```python
from build123d import *

# Parameters (mm, degrees)
FILLET1_R           = 1
SKETCH3_R           = 5.5
CUT_EXTRUDE1_DEPTH  = 0.35
CUT_EXTRUDE2_DEPTH  = 5
BOSS_EXTRUDE2_DEPTH = 2
SKETCH5_R           = 0.65
CUT_EXTRUDE3_DEPTH  = 5
SKETCH7_R           = 1.1
CUT_EXTRUDE4_DEPTH  = 8


with BuildPart() as part:
    # Sketch1 → Revolve1 (revolve)
    with BuildSketch(Plane.XY, mode=Mode.PRIVATE) as revolve1_sk:
        Polygon((-17.325922144, -3.94739572), (34.674077856, -3.94739572), (34.674077856, -4.54739572), (-17.825922144, -4.54739572), (-18.531230067, -0.94739572), (-18.531230067, 0.05260428), (-18.031230067, 0.05260428), align=None)
    revolve(revolve1_sk.sketch.rotate(Axis((-18.92728318, 4.55260428, 0), (1, 0, 0)), 270), axis=Axis((-18.92728318, 4.55260428, 0), (1, 0, 0)))

    # Fillet1
    fillet1_edges = [part.edges().sort_by_distance(p)[0] for p in [
        (-17.825922144, 4.55260428, -9.1),
    ]]
    fillet(fillet1_edges, radius=FILLET1_R)

    # Sketch3 → Cut-Extrude1 (cut)
    with BuildSketch(Plane.ZY.offset(18.531230067)):
        with Locations((0, 4.55260428)):
            Circle(SKETCH3_R)
    extrude(amount=-CUT_EXTRUDE1_DEPTH, mode=Mode.SUBTRACT)

    # Sketch4 → Cut-Extrude2 (cut)
    with BuildSketch(Plane(origin=(34.674077856, 0, 0), x_dir=(0, 0, -1), z_dir=(1, 0, 0))):
        Polygon((-13.628095951, 5.995190129), (5.056342646, -9.067736356), (14.470671699, 2.610037767), (-4.213766898, 17.672964252), align=None)
    extrude(amount=-CUT_EXTRUDE2_DEPTH, mode=Mode.SUBTRACT)

    # Sketch6 → Boss-Extrude2 (add)
    with BuildSketch(Plane(origin=(34.674077856, 0, 0), x_dir=(0, 0, -1), z_dir=(1, 0, 0))):
        Polygon((-6.25, -0.283182158), (-4.835786438, -1.69739572), (-6.25, -3.111609282), (-7.664213562, -1.69739572), align=None)
        Polygon((4.835786438, 10.80260428), (6.25, 12.216817842), (7.664213562, 10.80260428), (6.25, 9.388390718), align=None)
    extrude(amount=-BOSS_EXTRUDE2_DEPTH)

    # Sketch5 → Cut-Extrude3 (cut)
    with BuildSketch(Plane(origin=(34.674077856, 0, 0), x_dir=(0, 0, -1), z_dir=(1, 0, 0))):
        with Locations((6.25, 10.80260428)):
            Circle(SKETCH5_R)
        with Locations((-6.25, -1.69739572)):
            Circle(SKETCH5_R)
    extrude(amount=-CUT_EXTRUDE3_DEPTH, mode=Mode.SUBTRACT)

    # Sketch7 → Cut-Extrude4 (cut)
    with BuildSketch(Plane.ZY.offset(-32.674077856)):
        with Locations((6.25, -1.69739572)):
            Circle(SKETCH7_R)
        with Locations((-6.25, 10.80260428)):
            Circle(SKETCH7_R)
    extrude(amount=CUT_EXTRUDE4_DEPTH, mode=Mode.SUBTRACT)


solid = part.part
```
CAD build for the part. Positions are in the model's coordinates, mm. A direction names the side the tool comes from. Round coordinates to 2 decimals unless told otherwise and drop trailing zeros. Write each loop counter-clockwise with the first axis right and the second up, starting at its lowest first coordinate (ties: lowest second). Pieces come first, ordered by that corner, then holes. Notation, with made-up numbers: (34, 32.5) - (76, 32.5) arc R10 ccw to (76, 37.5) - close; hole circle Ø1 at (11.5, 76.5). An arc over 180 degrees is marked (long way). Return JSON: item names as keys, results as strings. Group by question number.
Item 1: Probe probe 1 along Y at (x, z) = (19, 0); probe 2 along Y at (x, z) = (29.5, -1); probe 3 along Z at (x, y) = (4, 7.5). List the from-to ranges inside material, lowest first.
Item 2: Band-saw the part on B-B on x = 11.5. List the corners of the cut face in (y, z), plus the area to 3 significant figures.
Item 3: Mould opens along X. For faces 1 (the face through (24.674, 11, -6)), 2 (the face through (33.69, -2.41, 6.95)), 3 (the face through (34.674, -1.9, 5.3)) say: +X half, -X half, draft (parallel to the pull), parting line (faces both ways), or undercut.
Item 4: 3-axis set-ups, long thin cutter, end or side, ignore diameter. For faces 4 (the face through (32.209, 13.239, -1.286)), 5 (the face through (-18.36, 9.19, 2.96)), 6 (the face through (24.674, -2, 6)): which of +Z, -Z, +X, -X, +Y, -Y reach the whole face in a straight line?
Item 5: Flat gauge pins, fed straight in: pin 1 Ø1.5 at (x, y) = (18.5, 0.5) entering from +Z; pin 2 Ø3 at (y, z) = (4.5, -2) entering from +X; pin 3 Ø3.5 at (y, z) = (10, 5.5) entering from +X; pin 4 Ø2.5 at (y, z) = (10, -6) entering from -X. Where does each tip first touch, or does it go through?
Item 6: Band-saw the part on A-A on x = 26.5. List the corners of the cut face in (y, z), plus the area to 3 significant figures.
Resolved:
{
 "1": {"probe 1": "y = -4.55 to -3.95, 13.05 to 13.65", "probe 2": "y = -4.49 to -3.89, 12.99 to 13.6", "probe 3": "z = -8.61 to -7.97, 7.97 to 8.61"},
 "2": {"outline": "circle Ø18.2 at (4.55, 0); hole circle Ø17 at (4.55, 0)", "area": "33.2 mm²"},
 "3": {"face 1": "undercut", "face 2": "draft", "face 3": "+X half"},
 "4": {"face 4": "+Z, +X, -Y", "face 5": "-X", "face 6": "none"},
 "5": {"pin 1": "stops at z = 8.48", "pin 2": "passes through", "pin 3": "stops at x = 29.67", "pin 4": "stops at x = -18.27"},
 "6": {"outline": "(-2.6, 5.62) arc R9.1 ccw to (10.18, -7.15) arc R1.1 cw to (9.79, -6.69) arc R8.5 cw to (-2.14, 5.24) arc R1.1 cw to start; (-1.07, 7.15) arc R1.1 cw to (-0.69, 6.69) arc R8.5 cw to (11.24, -5.24) arc R1.1 cw to (11.71, -5.62) arc R9.1 ccw to start", "area": "30.6 mm²"}
}
